```python
from build123d import *

# Parameters (mm, degrees)
SKETCH_1_R          = 4.25
EXTRUDE_1_DEPTH     = 1.8
SKETCH_2_R          = 2.5
SKETCH_2_R_2        = 2.05
EXTRUDE_2_DEPTH     = 22
FILLET_1_R          = 0.2
CUT_EXTRUDE_1_DEPTH = 1.5


with BuildPart() as part:
    # 草图1 → 凸台-拉伸1 (new body)
    with BuildSketch(Plane.XY):
        Circle(SKETCH_1_R)
    extrude(amount=EXTRUDE_1_DEPTH)

    # 草图2 → 凸台-拉伸2 (add)
    with BuildSketch(Plane.XY.offset(1.8)):
        Circle(SKETCH_2_R)
        Circle(SKETCH_2_R_2, mode=Mode.SUBTRACT)
    extrude(amount=EXTRUDE_2_DEPTH)

    # 圆角1
    fillet_1_edges = [part.edges().sort_by_distance(p)[0] for p in [
        (-4.25, 0, 0),
        (-4.25, 0, 1.8),
    ]]
    fillet(fillet_1_edges, radius=FILLET_1_R)

    # 草图3 → 切除-拉伸1 (cut)
    with BuildSketch(Plane(origin=(0, 0, 0), x_dir=(-1, 0, 0), z_dir=(0, 0, -1))):
        Polygon((1.443375673, 0), (0.721687836, 1.25), (-0.721687836, 1.25), (-1.443375673, 0), (-0.721687836, -1.25), (0.721687836, -1.25), align=None)
    extrude(amount=-CUT_EXTRUDE_1_DEPTH, mode=Mode.SUBTRACT)


solid = part.part
```
Verification items for the finished model (mm, model axes). A direction names the side the tool comes from. Coordinates: 2 decimals unless noted, no trailing zeros. Write each loop counter-clockwise with the first axis right and the second up, starting at its lowest first coordinate (ties: lowest second). Pieces come first, ordered by that corner, then holes. Notation, with made-up numbers: (-7, 10) - (9, 10) arc R8 cw to (9, 23) - close; hole circle Ø9 at (79.25, 34.5). An arc over 180 degrees is marked (long way). Write item = value, one per line.
Q1. Go/stop test with flat-tipped pins: pin 1 Ø4 at (y, z) = (2.5, 6.5) entering from -X; pin 2 Ø1 at (y, z) = (0, 12) entering from -X; pin 3 Ø0.7 at (x, z) = (-0.5, 0.5) entering from -Y. Record where each tip stops, or that it passes through.
Answer:
pin_1 = -2.45
pin_2 = -2.5
pin_3 = -4.25
Q2. Access from +Z, -Z, +X, -X, +Y, -Y to the whole of each face (thin tool, end or side, straight path). Record for faces 1 (the face through (0, -2, 0)), 2 (the face through (-1.08, -0.63, 0.74)), 3 (the face through (-0.54, -2.44, 12.65)).
Answer:
face_1 = -Z, +X, -X, +Y, -Y
face_2 = -Z
face_3 = +Z
Q3. Cross-section at B-B (z = 18.5). Enter the section's corners in (x, y).
Answer:
outline = circle Ø5 at (0, 0); hole circle Ø4.1 at (0, 0)
Q4. Material ranges on L1, parallel to Y at x = 0, z = 13.25; L2, parallel to Z at x = -2, y = 0; L3, parallel to X at y = -1.75, z = 12.75, recorded low to high. Write a range as from..to.
Answer:
L1 = -2.5..-2.05, 2.05..2.5
L2 = 0..1.8
L3 = -1.79..-1.07, 1.07..1.79
Q5. Cross-section at A-A (x = 0). Enter the section's corners in (y, z).
Answer:
outline = (-4.25, 0.2) arc R0.2 ccw to (-4.05, 0) - (-1.25, 0) - (-1.25, 1.5) - (1.25, 1.5) - (1.25, 0) - (4.05, 0) arc R0.2 ccw to (4.25, 0.2) - (4.25, 1.6) arc R0.2 ccw to (4.05, 1.8) - (2.5, 1.8) - (2.5, 23.8) - (2.05, 23.8) - (2.05, 1.8) - (-2.05, 1.8) - (-2.05, 23.8) - (-2.5, 23.8) - (-2.5, 1.8) - (-4.05, 1.8) arc R0.2 ccw to (-4.25, 1.6) - close
Q6. Mould release check, pull along X, two halves, no side actions. Record for faces 4 (the face through (1.088, -0.616, 0.74)), 5 (the face through (2.285, 3.584, 0.89)), 6 (the face through (2, 2, 1.8)): released by +X, released by -X, zero draft, split by the parting line, or undercut.
Answer:
face_4 = undercut
face_5 = split by the parting line
face_6 = zero draft
